Check sheet for the modelled part. Datum: model origin and axes. Units: mm. Face numbers are marked on the shaded views. A direction names the side the tool comes from. Coordinates: 2 decimals unless noted, no trailing zeros. Write each loop counter-clockwise with the first axis right and the second up, starting at its lowest first coordinate (ties: lowest second). Pieces come first, ordered by that corner, then holes. Notation, with made-up numbers: (43, 52.5) - (100, 52.5) arc R32 ccw to (100, 87.5) - close; hole circle Ø4 at (17, 42). An arc over 180 degrees is marked (long way). Answer as CSV lines item,"result". Start each with the question number.
from build123d import *

# Parameters (mm, degrees)
F1_DEPTH = 60.325
F2_R     = 8.001
F3_DEPTH = 25.4
F4_R     = 3.175
F5_DEPTH = 25.4


with BuildPart() as f1:
    # F0 (on Front) → F1 (new body)
    with BuildSketch(Plane.XZ):
        with BuildLine():
            Line((-4.7625, 3.175), (-69.85, 3.175))
            Line((-69.85, 3.175), (-69.85, 0))
            Line((-69.85, 0), (-4.7625, 0))
            ThreePointArc((-4.7625, 0), (-1.394904, 1.394904), (0, 4.7625))
            Line((0, 4.7625), (0, 73.3425))
            ThreePointArc((0, 73.3425), (0.464968, 74.465032), (1.5875, 74.93))
            Line((1.5875, 74.93), (45.72, 74.93))
            Line((45.72, 74.93), (45.72, 78.105))
            Line((45.72, 78.105), (1.5875, 78.105))
            ThreePointArc((1.5875, 78.105), (-1.780096, 76.710096), (-3.175, 73.3425))
            Line((-3.175, 73.3425), (-3.175, 4.7625))
            ThreePointArc((-3.175, 4.7625), (-3.639968, 3.639968), (-4.7625, 3.175))
        make_face()
    extrude(amount=F1_DEPTH)

    # F2 (on face) → F3 (cut)
    with BuildSketch(Plane.XY.offset(78.105)):
        with Locations((34.29, -12.7)):
            Circle(F2_R)
        with Locations((34.29, -47.625)):
            Circle(F2_R)
    extrude(amount=-F3_DEPTH, mode=Mode.SUBTRACT)

    # F4 (on face) → F5 (cut)
    with BuildSketch(Plane.XY.offset(3.175)):
        with Locations((-57.15, -12.7)):
            Circle(F4_R)
        with Locations((-17.4625, -12.7)):
            Circle(F4_R)
        with Locations((-17.4625, -47.625)):
            Circle(F4_R)
        with Locations((-57.15, -47.625)):
            Circle(F4_R)
    extrude(amount=-F5_DEPTH, mode=Mode.SUBTRACT)


solid = f1.part
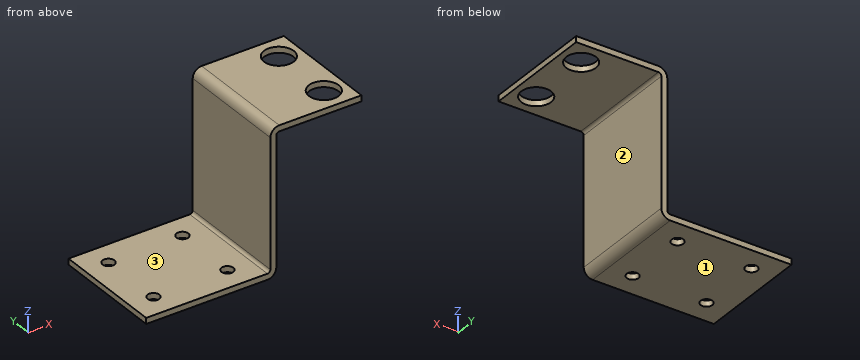
(1) Cross-section at B-B on y = -12.7. State how many separate pieces and enclosed holes the cut face has, plus the area to 3 significant figures.
(2) Go/stop test with flat-tipped pins: P1, Ø12, axis at y = -23.5, z = 67.5, coming from the +X side; P2, Ø18.5, axis at x = 34.29, y = -12.7, coming from the +Z side (3 decimals); P3, Ø22, axis at x = 18.5, y = -38, coming from the -Z side; P4, Ø10, axis at x = -57.15, y = -47.625, coming from the +Z side (3 decimals). Record where each tip stops, or that it passes through.
(3) Cross-section at D-D on x = 34.29. Record the boundary of the cut face in (y, z) (3 decimals), plus the area to 3 significant figures.
(4) Tool access check on the marked faces 1, 2 and 3. Record the directions out of +Z, -Z, +X, -X, +Y, -Y that give a thin tool (end or side, any length) a straight path to the whole face; none if there is none.
(5) Cross-section at A-A on x = -57.15. Record the boundary of the cut face in (y, z) (3 decimals), plus the area to 3 significant figures.
(6) Material ranges on probe 1 along Y at (x, z) = (34, 76) (3 decimals); probe 2 along X at (y, z) = (-49.5, 43) (3 decimals); probe 3 along Z at (x, y) = (-17, -42) (3 decimals), recorded low to high. Write a range as from..to.
Checked values:
1,separate pieces,"4"
1,enclosed holes,"0"
1,area,"505 mm^2"
2,P1,"x = 0.01"
2,P2,"z = 78.105"
2,P3,"z = 74.93"
2,P4,"z = 3.175"
3,outline,"(-60.325, 74.93) - (-55.626, 74.93) - (-55.626, 78.105) - (-60.325, 78.105) - close; (-39.624, 74.93) - (-20.701, 74.93) - (-20.701, 78.105) - (-39.624, 78.105) - close; (-4.699, 74.93) - (0, 74.93) - (0, 78.105) - (-4.699, 78.105) - close"
3,area,"89.9 mm^2"
4,face 1,"-Z, +X, -X, +Y, -Y"
4,face 2,"-Z, +X, +Y, -Y"
4,face 3,"+Z, -X, +Y, -Y"
5,outline,"(-60.325, 0) - (-50.8, 0) - (-50.8, 3.175) - (-60.325, 3.175) - close; (-44.45, 0) - (-15.875, 0) - (-15.875, 3.175) - (-44.45, 3.175) - close; (-9.525, 0) - (0, 0) - (0, 3.175) - (-9.525, 3.175) - close"
5,area,"151 mm^2"
6,probe 1,"-60.325..-55.621, -39.629..-20.696, -4.704..0"
6,probe 2,"-3.175..0"
6,probe 3,"0..3.175"
